from build123d import *

# Parameters (mm, degrees)
SKETCH1_W           = 103
SKETCH1_H           = 63.711340206
SKETCH1_R           = 1.75
SKETCH1_W_2         = 16
SKETCH1_H_2         = 3.2
SKETCH1_W_3         = 3.2
SKETCH1_H_3         = 11.2
SKETCH1_H_4         = 16
BOSS_EXTRUDE1_DEPTH = 3
FILLET1_R           = 5


with BuildPart() as part:
    # Sketch1 → Boss-Extrude1 (new body)
    with BuildSketch(Plane(origin=(0, 0, 0), x_dir=(1, 0, 0), z_dir=(0, 1, 0))):
        Rectangle(SKETCH1_W, SKETCH1_H)
        with Locations(Location((-42.5, 24.25, 0), (0, 0, 270))):
            Circle(SKETCH1_R, mode=Mode.SUBTRACT)
        with Locations(Location((42.5, 24.25, 0), (0, 0, 270))):
            Circle(SKETCH1_R, mode=Mode.SUBTRACT)
        with Locations(Location((-42.5, -24.25, 0), (0, 0, 270))):
            Circle(SKETCH1_R, mode=Mode.SUBTRACT)
        with Locations(Location((42.5, -24.25, 0), (0, 0, 270))):
            Circle(SKETCH1_R, mode=Mode.SUBTRACT)
        with Locations((-28, 28.4)):
            Rectangle(SKETCH1_W_2, SKETCH1_H_2, mode=Mode.SUBTRACT)
        with Locations((28, 28.4)):
            Rectangle(SKETCH1_W_2, SKETCH1_H_2, mode=Mode.SUBTRACT)
        with Locations((-46.9, 16.475)):
            Rectangle(SKETCH1_W_3, SKETCH1_H_3, mode=Mode.SUBTRACT)
        with Locations((-46.9, -16.475)):
            Rectangle(SKETCH1_W_3, SKETCH1_H_3, mode=Mode.SUBTRACT)
        with Locations((0, 28.4)):
            Rectangle(SKETCH1_W_2, SKETCH1_H_2, mode=Mode.SUBTRACT)
        with Locations((-28, -28.4)):
            Rectangle(SKETCH1_W_2, SKETCH1_H_2, mode=Mode.SUBTRACT)
        with Locations((28, -28.4)):
            Rectangle(SKETCH1_W_2, SKETCH1_H_2, mode=Mode.SUBTRACT)
        with Locations((0, -28.4)):
            Rectangle(SKETCH1_W_2, SKETCH1_H_2, mode=Mode.SUBTRACT)
        with Locations((46.9, -14)):
            Rectangle(SKETCH1_W_3, SKETCH1_H_4, mode=Mode.SUBTRACT)
        with Locations((46.9, 14)):
            Rectangle(SKETCH1_W_3, SKETCH1_H_4, mode=Mode.SUBTRACT)
    extrude(amount=BOSS_EXTRUDE1_DEPTH)

    # Fillet1
    fillet1_edges = [part.edges().sort_by_distance(p)[0] for p in [
        (51.5, 1.5, 31.855670103),
        (-51.5, 1.5, 31.855670103),
        (-51.5, 1.5, -31.855670103),
        (51.5, 1.5, -31.855670103),
    ]]
    fillet(fillet1_edges, radius=FILLET1_R)


solid = part.part
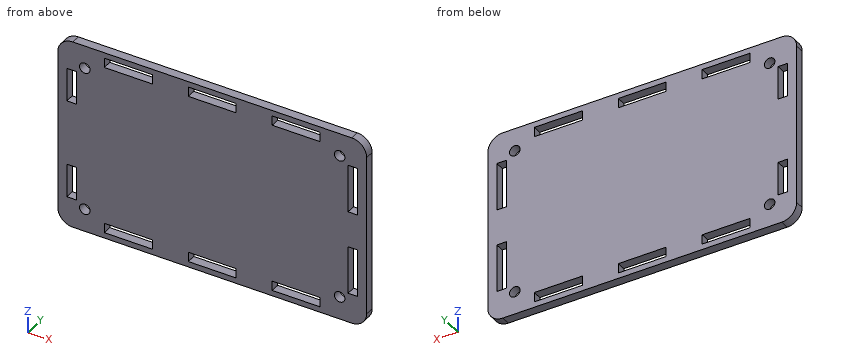
Read the model definition and answer for the solid it produces. Units are mm, in the model's axes. Coordinates: 2 decimals unless noted, no trailing zeros. Loops run counter-clockwise (first coordinate to the right, second up) from the corner with the lowest first, then second, coordinate; pieces in that order, holes last.
Q1. Each of these flat-tipped pins is pushed along its axis until it touches: pin 1 Ø1.5 at (y, z) = (1.5, -28) entering from +X; pin 2 Ø2 at (x, z) = (42.5, 24.25) entering from +Y; pin 3 Ø1.5 at (y, z) = (2, -28) entering from -X. Where does it stop, or does it pass through?
Q2. The part is cut by section C-C on z = 24.25. Write down the section's boundary in (x, y), and give its area (3 significant figures).
Q3. Consider probe 1 along X at (y, z) = (1.85, -20); probe 2 along X at (y, z) = (1.4, 24.25); probe 3 along Z at (x, y) = (-31, 0.3). Determine where each line is inside the solid, lowest interval first.
Q4. The part is cut by section D-D on y = 1.6. Give the number of separate pieces and of enclosed holes in the cut face, and give its area (3 significant figures).
Q5. The part is cut by section A-A on z = -7. Write down the section's boundary in (x, y).
Q6. The part is cut by section B-B on x = -42.5. Write down the section's boundary in (y, z).
Results below:
1. pin 1: stops at x = 51.48
1. pin 2: passes through
1. pin 3: stops at x = -51.48
2. outline: (-51.5, 0) - (-44.25, 0) - (-44.25, 3) - (-51.5, 3) - close; (-40.75, 0) - (40.75, 0) - (40.75, 3) - (-40.75, 3) - close; (44.25, 0) - (51.5, 0) - (51.5, 3) - (44.25, 3) - close
2. area: 288 mm2
3. probe 1: x = -51.5 to -48.5, -45.3 to 45.3, 48.5 to 51.5
3. probe 2: x = -51.5 to -44.25, -40.75 to 40.75, 44.25 to 51.5
3. probe 3: z = -31.86 to -30, -26.8 to 26.8, 30 to 31.86
4. separate pieces: 1
4. enclosed holes: 14
4. area: 6,020 mm2
5. outline: (-51.5, 0) - (45.3, 0) - (45.3, 3) - (-51.5, 3) - close; (48.5, 0) - (51.5, 0) - (51.5, 3) - (48.5, 3) - close
6. outline: (0, -31.86) - (3, -31.86) - (3, -26) - (0, -26) - close; (0, -22.5) - (3, -22.5) - (3, 22.5) - (0, 22.5) - close; (0, 26) - (3, 26) - (3, 31.86) - (0, 31.86) - close
